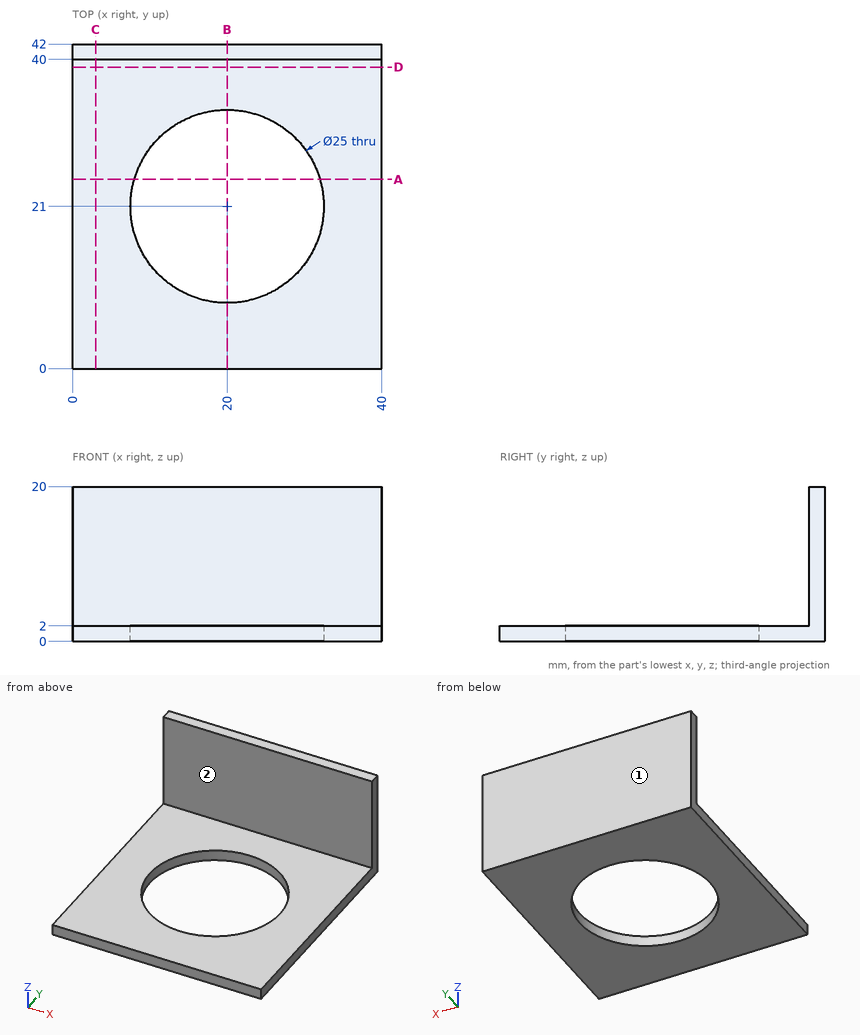
The drawing under review shows one solid part. Ordinate dimensions are in mm from its lowest x, y, z. A direction names the side the tool comes from. Round coordinates to 2 decimals unless told otherwise and drop trailing zeros. Loops run counter-clockwise (first coordinate to the right, second up) from the corner with the lowest first, then second, coordinate; pieces in that order, holes last. Notation, with made-up numbers: (57.25, -22) - (100.25, -22) arc R20 ccw to (100.25, 11) - close; hole circle Ø8 at (35, 47.25). An arc over 180 degrees is marked (long way). Use one line per item in the form item = value.
Item 1: Consider section D-D on y = 39. Write out the cut boundary in (x, z).
Answers:
outline = (0, 0) - (40, 0) - (40, 2) - (0, 2) - close
Item 2: Consider section A-A on y = 24.5. Write out the cut boundary in (x, z), then the cut area to 3 significant figures.
Answers:
outline = (0, 0) - (8, 0) - (8, 2) - (0, 2) - close; (32, 0) - (40, 0) - (40, 2) - (32, 2) - close
area = 32.0 mm^2
Item 3: For line 1 (Y direction, x = 20, z = 0.65); line 2 (Y direction, x = 19, z = 5.75); line 3 (Z direction, x = 26, y = 34), list the stretches that pass through material, from the lowest coordinate up.
Answers:
line_1 = 0 to 8.5, 33.5 to 42
line_2 = 40 to 42
line_3 = 0 to 2
Item 4: Consider section C-C on x = 3. Write out the cut boundary in (y, z).
Answers:
outline = (0, 0) - (42, 0) - (42, 20) - (40, 20) - (40, 2) - (0, 2) - close
Item 5: Consider section B-B on x = 20. Write out the cut boundary in (y, z).
Answers:
outline = (0, 0) - (8.5, 0) - (8.5, 2) - (0, 2) - close; (33.5, 0) - (42, 0) - (42, 20) - (40, 20) - (40, 2) - (33.5, 2) - close
Item 6: Clearance check with flat-ended pins moving along their axes: P1, Ø6, axis at x = 5, z = 5.5, coming from the -Y side; P2, Ø22.5, axis at x = 20, y = 21, coming from the -Z side; P3, Ø20, axis at x = 25.5, y = 14.5, coming from the +Z side. State where each tip first meets the part, or that it passes through.
Answers:
P1 = 40
P2 = through
P3 = 2
Item 7: Tool access review of the marked faces 1 and 2: name each direction out of +Z, -Z, +X, -X, +Y, -Y from which nothing blocks a thin tool from reaching the whole face with its end or side.
Answers:
face_1 = +Z, -Z, +X, -X, +Y
face_2 = +Z, +X, -X, -Y
